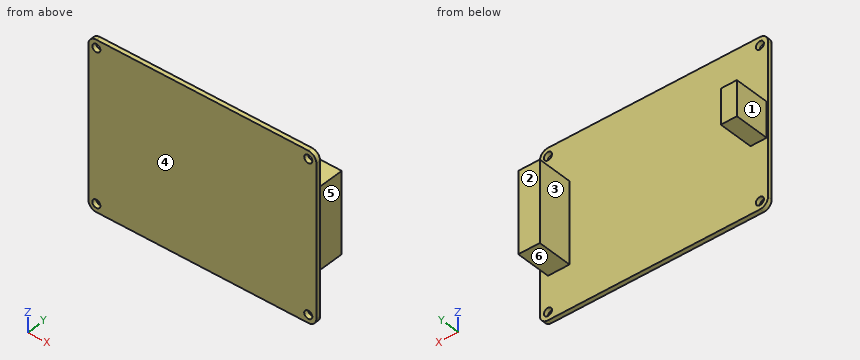
from build123d import *

# Parameters (mm, degrees)
SKETCH1_W           = 84.8
SKETCH1_H           = 62
SKETCH1_R           = 1.5
BOSS_EXTRUDE1_DEPTH = 1.65
FILLET1_R           = 3
SKETCH2_W           = 6
SKETCH2_H           = 13
SKETCH2_W_2         = 8
SKETCH2_H_2         = 30
BOSS_EXTRUDE2_DEPTH = 13


with BuildPart() as part:
    # Sketch1 → Boss-Extrude1 (new body)
    with BuildSketch(Plane(origin=(0, 0, 0), x_dir=(1, 0, 0), z_dir=(0, 1, 0))):
        Rectangle(SKETCH1_W, SKETCH1_H)
        with Locations((-39.4, 28)):
            Circle(SKETCH1_R, mode=Mode.SUBTRACT)
        with Locations((39.4, 28)):
            Circle(SKETCH1_R, mode=Mode.SUBTRACT)
        with Locations((39.4, -28)):
            Circle(SKETCH1_R, mode=Mode.SUBTRACT)
        with Locations((-39.4, -28)):
            Circle(SKETCH1_R, mode=Mode.SUBTRACT)
    extrude(amount=BOSS_EXTRUDE1_DEPTH)

    # Fillet1
    fillet1_edges = [part.edges().sort_by_distance(p)[0] for p in [
        (-42.4, 0.825, -31),
        (42.4, 0.825, -31),
        (42.4, 0.825, 31),
        (-42.4, 0.825, 31),
    ]]
    fillet(fillet1_edges, radius=FILLET1_R)

    # Sketch2 → Boss-Extrude2 (add)
    with BuildSketch(Plane(origin=(0, 1.65, 0), x_dir=(1, 0, 0), z_dir=(0, 1, 0))):
        with Locations((-38.9, 0)):
            Rectangle(SKETCH2_W, SKETCH2_H)
        with Locations((35.4, 0)):
            Rectangle(SKETCH2_W_2, SKETCH2_H_2)
    extrude(amount=BOSS_EXTRUDE2_DEPTH)


solid = part.part
For this review, take the finished solid that the model builds, in its own axes (mm). Face numbers are marked on the shaded views. A direction names the side the tool comes from. Give positions to 0.01 mm unless a question says otherwise; leave off trailing zeros. Loops run counter-clockwise (first coordinate to the right, second up) from the corner with the lowest first, then second, coordinate; pieces in that order, holes last. Notation, with made-up numbers: M 28,-2.5 L 53,-2.5 A14 cw 53,18.5 Z; hole C -21.5,35 d8. An arc over 180 degrees is marked long. Put each result on its own line as item: value. Start each with the question number.
(1) For pin 1 (6.5 mm diameter, centred on x = 35.5, y = 7.5, fed in from -Z); pin 2 (3 mm diameter, centred on y = 12, z = 10, fed in from +X); pin 3 (5 mm diameter, centred on x = -39.4, z = 28, fed in from +Y); pin 4 (2.5 mm diameter, centred on x = -39.4, z = -28, fed in from +Y), all flat-tipped, find the tip position at first contact; note any pin that passes through.
(2) Machinability: for the marked faces 4, 5 and 6, which of the approach directions +Z, -Z, +X, -X, +Y, -Y give a long, thin tool a straight path to every point of the face, cutting with its end or side? Answer none if there is none.
(3) The part is to be moulded in two halves that separate along X. For the marked faces 1, 2 and 3, say which applies: +X half, -X half, draft (parallel to the pull), parting line (faces both ways), or undercut.
(4) Wall thickness on L1, parallel to Z at x = -39.4, y = 0.45; L2, parallel to X at y = 1.1, z = 28; L3, parallel to Y at x = 1.5, z = 16.5: over which ranges is each line inside the solid? List them lowest first.
(5) Add section B-B, the plane x = 24. Write out the cut boundary in (y, z).
(6) Add section A-A, the plane y = 9.5. Write out the cut boundary in (x, z).
(7) Add section C-C, the plane z = 17.5. Write out the cut boundary in (x, y).
Result:
1. pin 1: stops at z = -15
1. pin 2: stops at x = 39.4
1. pin 3: stops at y = 1.65
1. pin 4: passes through
2. face 4: +Z, -Z, +X, -X, -Y
2. face 5: +Z, -Z, +X, +Y
2. face 6: -Z, +X, -X, +Y
3. face 1: -X half
3. face 2: draft
3. face 3: undercut
4. L1: z = -31 to -29.5, -26.5 to 26.5, 29.5 to 31
4. L2: x = -42.4 to -40.9, -37.9 to 37.9, 40.9 to 42.4
4. L3: y = 0 to 1.65
5. outline: M 0,-31 L 1.65,-31 L 1.65,31 L 0,31 Z
6. outline: M -41.9,-6.5 L -35.9,-6.5 L -35.9,6.5 L -41.9,6.5 Z; M 31.4,-15 L 39.4,-15 L 39.4,15 L 31.4,15 Z
7. outline: M -42.4,0 L 42.4,0 L 42.4,1.65 L -42.4,1.65 Z
